from build123d import *

# Parameters (mm, degrees)
SKETCH1_W           = 15.875
SKETCH1_H           = 15.875
BASE_EXTRUDE_DEPTH  = 3.175
SHELL1_T            = -1.5875
SKETCH4_R           = 1.27
BOSS_EXTRUDE2_DEPTH = 1.5875
CUT_EXTRUDE2_START  = -1.5875
SKETCH5_R           = 0.635
CUT_EXTRUDE2_DEPTH  = 1.5875
FILLET1_R           = 0.254


with BuildPart() as part:
    # Sketch1 → Base-Extrude (new body)
    with BuildSketch(Plane(origin=(0, 0, 0), x_dir=(1, 0, 0), z_dir=(0, 1, 0))):
        Rectangle(SKETCH1_W, SKETCH1_H)
    extrude(amount=BASE_EXTRUDE_DEPTH)

    # Shell1
    shell1_openings = [part.faces().sort_by_distance(p)[0] for p in [
        (0, 0, 0),
    ]]
    offset(amount=SHELL1_T, openings=shell1_openings, kind=Kind.INTERSECTION)

    # Sketch4 → Boss-Extrude2 (add)
    with BuildSketch(Plane.XZ.offset(-1.5875)):
        with Locations(Location((-3.81, 0, 0), (0, 0, 90))):
            Circle(SKETCH4_R)
        with Locations(Location((0, 3.81, 0), (0, 0, 90))):
            Circle(SKETCH4_R)
    extrude(amount=BOSS_EXTRUDE2_DEPTH)

    # Sketch5 → Cut-Extrude2 (cut)
    with BuildSketch(Plane.XZ.offset(CUT_EXTRUDE2_START)):
        with Locations(Location((0, 3.81, 0), (0, 0, 270))):
            Circle(SKETCH5_R)
        with Locations(Location((-3.81, 0, 0), (0, 0, 270))):
            Circle(SKETCH5_R)
    extrude(amount=CUT_EXTRUDE2_DEPTH, mode=Mode.SUBTRACT)

    # Fillet1
    fillet1_edges = [part.edges().sort_by_distance(p)[0] for p in [
        (7.9375, 3.175, 0),
        (0, 3.175, -7.9375),
        (-7.9375, 3.175, 0),
        (0, 3.175, 7.9375),
    ]]
    fillet(fillet1_edges, radius=FILLET1_R)


solid = part.part
Input: part model. Units: mm. Frame: model coordinates. A direction names the side the tool comes from. Give positions to 0.01 mm unless a question says otherwise; leave off trailing zeros. Answer as a JSON object with one key per item and string values. Group by question number.
Q1. Cut plane A-A, the plane y = 0.65. Count the separate pieces of the cut face and the enclosed holes in it, then the cut area to 3 significant figures.
Q2. First-contact query: pin 1 Ø8 at (x, z) = (-1.5, -6.5) entering from -Y; pin 2 Ø1 at (x, z) = (-1.5, 1.5) entering from -Y. Flat tips, straight axial feed; report the tip coordinate or a pass-through.
Q3. Set-up query: faces 1 (the face through (-7.938, 1, 0)), 2 (the face through (0.191, 0.805, 3.204)). Return all of +Z, -Z, +X, -X, +Y, -Y with unobstructed straight access to the full face (end or side cutting, diameter ignored); none if empty.
Q4. Mould query, pull axis Z, two halves, no side actions, for faces 3 (the face through (0, 1, 7.938)), 4 (the face through (7.938, 1, 0)), 5 (the face through (0, 1, -6.35)), 6 (the face through (0, 1.588, 4)). Classes: pulls with the +Z half, pulls with the -Z half, needs draft (parallel to the pull), parting line crosses it, or undercut.
Q5. Line query: probe 1 along X at (y, z) = (0.55, -5.5). Output: solid intervals per line, ascending.
Results:
{
 "1": {"separate pieces": "3", "enclosed holes": "3", "area": "98.3 mm^2"},
 "2": {"pin 1": "y = 0", "pin 2": "y = 1.59"},
 "3": {"face 1": "+Z, -Z, -X, +Y, -Y", "face 2": "-Y"},
 "4": {"face 3": "pulls with the +Z half", "face 4": "needs draft", "face 5": "undercut", "face 6": "undercut"},
 "5": {"probe 1": "-7.94 to -6.35, 6.35 to 7.94"}
}
